Geometry check sheet. Reference: the model listing, model coordinates, mm. A direction names the side the tool comes from. Give positions to 0.01 mm unless a question says otherwise; leave off trailing zeros. Loops run counter-clockwise (first coordinate to the right, second up) from the corner with the lowest first, then second, coordinate; pieces in that order, holes last. Notation, with made-up numbers: (-34, 54.5) -> (-30, 54.5) arc R24 ccw to (-30, 86.5) -> close; hole circle Ø9 at (50.25, 62.25). An arc over 180 degrees is marked (long way). Answer as a JSON object with one key per item and string values.
from build123d import *

# Parameters (mm, degrees)
SKETCH_1_W          = 20
SKETCH_1_H          = 9
SKETCH_1_R          = 1.05
EXTRUDE_1_DEPTH     = 3
SKETCH_2_W          = 20
SKETCH_2_H          = 3
EXTRUDE_2_DEPTH     = 5
SKETCH_3_R          = 1.05
CUT_EXTRUDE_1_DEPTH = 10
FILLET_1_R          = 3
FILLET_2_R          = 3
FILLET_3_R          = 2
FILLET_4_R          = 2
FILLET_7_R          = 1
FILLET_8_R          = 1


with BuildPart() as part:
    # 草图1 → 凸台-拉伸1 (new body)
    with BuildSketch(Plane(origin=(0, 0, 0), x_dir=(0, 0, -1), z_dir=(1, 0, 0))):
        with Locations((10, -4.5)):
            Rectangle(SKETCH_1_W, SKETCH_1_H)
        with Locations((3.37, -2)):
            Circle(SKETCH_1_R, mode=Mode.SUBTRACT)
        with Locations(Location((16.63, -2, 0), (0, 0, 180))):
            Circle(SKETCH_1_R, mode=Mode.SUBTRACT)
    extrude(amount=EXTRUDE_1_DEPTH)

    # 草图2 → 凸台-拉伸2 (add)
    with BuildSketch(Plane(origin=(3, 0, 0), x_dir=(0, 0, -1), z_dir=(1, 0, 0))):
        with Locations((10, -7.5)):
            Rectangle(SKETCH_2_W, SKETCH_2_H)
    extrude(amount=EXTRUDE_2_DEPTH)

    # 草图3 → 切除-拉伸1 (cut)
    with BuildSketch(Plane(origin=(8, 0, 0), x_dir=(0, 0, -1), z_dir=(1, 0, 0))):
        with Locations((3.37, -7.5)):
            Circle(SKETCH_3_R)
        with Locations((16.63, -7.5)):
            Circle(SKETCH_3_R)
    extrude(amount=-CUT_EXTRUDE_1_DEPTH, mode=Mode.SUBTRACT)

    # 圆角1
    fillet_1_edges = [part.edges().sort_by_distance(p)[0] for p in [
        (1.5, 0, 0),
    ]]
    fillet(fillet_1_edges, radius=FILLET_1_R)

    # 圆角2
    fillet_2_edges = [part.edges().sort_by_distance(p)[0] for p in [
        (1.5, 0, -20),
    ]]
    fillet(fillet_2_edges, radius=FILLET_2_R)

    # 圆角3
    fillet_3_edges = [part.edges().sort_by_distance(p)[0] for p in [
        (4, -9, -20),
    ]]
    fillet(fillet_3_edges, radius=FILLET_3_R)

    # 圆角4
    fillet_4_edges = [part.edges().sort_by_distance(p)[0] for p in [
        (4, -9, 0),
    ]]
    fillet(fillet_4_edges, radius=FILLET_4_R)

    # 圆角7
    fillet_7_edges = [part.edges().sort_by_distance(p)[0] for p in [
        (5.5, -6, 0),
    ]]
    fillet(fillet_7_edges, radius=FILLET_7_R - 0.0001)  # a hair under: the kernel refuses the full size

    # 圆角8
    fillet_8_edges = [part.edges().sort_by_distance(p)[0] for p in [
        (5.5, -6, -20),
    ]]
    fillet(fillet_8_edges, radius=FILLET_8_R - 0.0001)  # a hair under: the kernel refuses the full size


solid = part.part
1) Section check A-A on z = -3.37. Record the cut outline in (x, y), plus the area to 3 significant figures.
Geometry check:
{"outline": "(0, -9) -> (8, -9) -> (8, -8.55) -> (0, -8.55) -> close; (0, -6.45) -> (8, -6.45) -> (8, -6) -> (3, -6) -> (3, -3.05) -> (0, -3.05) -> close; (0, -0.95) -> (3, -0.95) -> (3, 0) -> (0, 0) -> close", "area": "18.9 mm2"}
2) Material ranges on line 1 along Y through (x, z) = (2.1, -3.37); line 2 along Z through (x, y) = (5.25, -8.25); line 3 along Y through (x, z) = (5.75, -3.37), recorded low to high. Write a range as from..to.
Geometry check:
{"line 1": "y = -9..-8.55, -6.45..-3.05, -0.95..0", "line 2": "z = -19.56..-17.36, -15.9..-4.1, -2.64..-0.44", "line 3": "y = -9..-8.55, -6.45..-6"}
3) Section check D-D on x = 2. Record the cut outline in (y, z).
Geometry check:
{"outline": "(-9, -18) arc R2 ccw to (-7, -20) -> (-3, -20) arc R3 ccw to (0, -17) -> (0, -3) arc R3 ccw to (-3, 0) -> (-7, 0) arc R2 ccw to (-9, -2) -> close; hole circle Ø2.1 at (-7.5, -16.63); hole circle Ø2.1 at (-7.5, -3.37); hole circle Ø2.1 at (-2, -16.63); hole circle Ø2.1 at (-2, -3.37)"}
4) Section check B-B on x = 3.5. Count the separate pieces of the cut face and the enclosed holes in it, plus the area to 3 significant figures.
Geometry check:
{"separate pieces": "1", "enclosed holes": "2", "area": "50.9 mm2"}
5) Draft check along Y on faces 4 (the face through (1, 0, -10)), 5 (the face through (4.06, -7.18, -17.63)), 6 (the face through (4, -9, -10)). Enter one of: pulls with the +Y half, pulls with the -Y half, needs draft (parallel to the pull), parting line crosses it, or undercut.
Geometry check:
{"face 4": "pulls with the +Y half", "face 5": "undercut", "face 6": "pulls with the -Y half"}
6) Depth check by flat-ended pin: P1, Ø3.5, axis at y = -2, z = -13, coming from the +X side; P2, Ø2.5, axis at x = 6, z = -7.5, coming from the +Y side. Enter the tip coordinate at first touch or a pass-through.
Geometry check:
{"P1": "stops at x = 3", "P2": "stops at y = -6"}
7) Tool access check on faces 1 (the face through (5.535, -6.301, -19.715)), 2 (the face through (5.535, -6.301, -0.285)), 3 (the face through (5, -6, -10)). Record the directions out of +Z, -Z, +X, -X, +Y, -Y that give a thin tool (end or side, any length) a straight path to the whole face; none if there is none.
Geometry check:
{"face 1": "-Z, +X, +Y", "face 2": "+Z, +X, +Y", "face 3": "+Z, -Z, +X, +Y"}
8) Section check C-C on y = -8. Record the cut outline in (x, z).
Geometry check:
{"outline": "(0, -19.73) -> (8, -19.73) -> (8, -17.55) -> (0, -17.55) -> close; (0, -15.71) -> (8, -15.71) -> (8, -4.29) -> (0, -4.29) -> close; (0, -2.45) -> (8, -2.45) -> (8, -0.27) -> (0, -0.27) -> close"}
